Here's the drawing with two shaded views (mm, measured from the low corner). I have some questions. Coordinates: 2 decimals unless noted, no trailing zeros. Order: outer loops, then holes, each group sorted by start corner. A loop starts at its lowest first (then second) coordinate and runs counter-clockwise, first axis right, second up. Notation, with made-up numbers: (77, 88.25) -> (90, 88.25) arc R15 cw to (90, 101.25) -> close; hole circle Ø7 at (80, -4). An arc over 180 degrees is marked (long way). One line per item, written item: value. Start each with the question number.
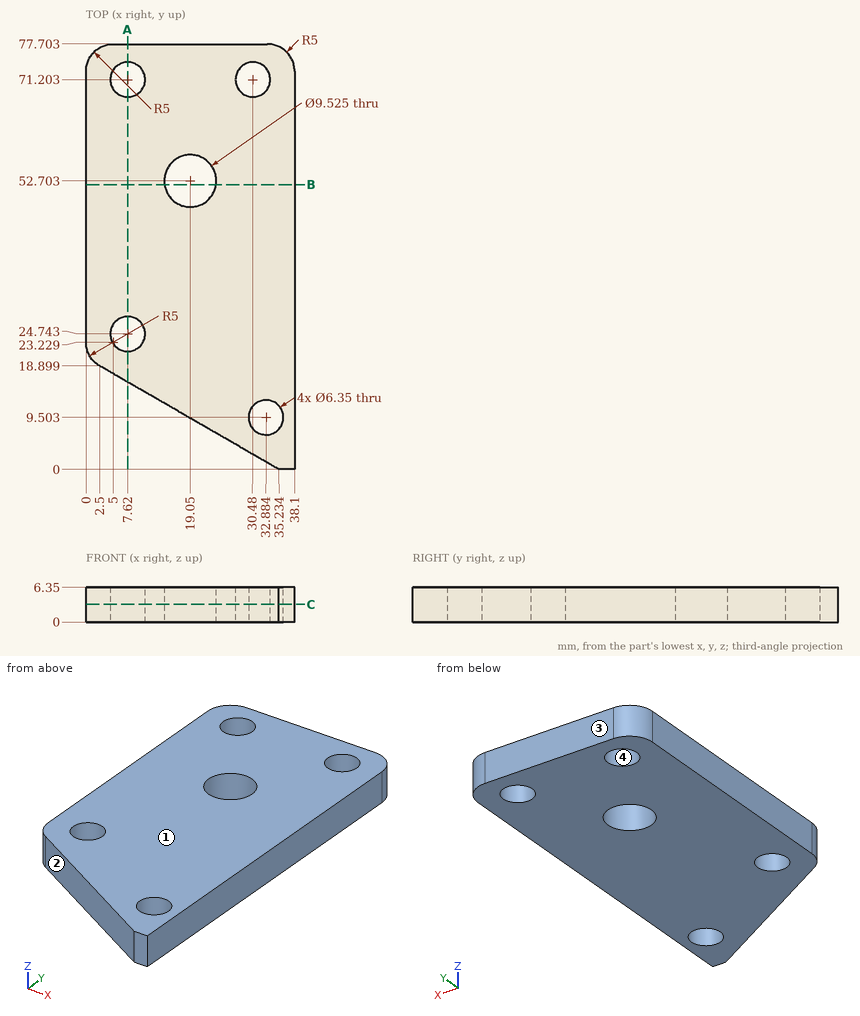
Q1. Imagine slicing it at C-C (z = 3.25). Count the separate pieces of the cut face and the enclosed holes in it, plus the area to 3 significant figures.
Q2. Imagine slicing it at A-A (x = 7.62). Write out the boundary of the cut face in (y, z).
Q3. I need wall thicknesses on line 1 (Y direction, x = 31, z = 1.5) (1 decimal); line 2 (Y direction, x = 7.62, z = 5); line 3 (X direction, y = 26, z = 5.25) (1 decimal). Which ranges of each line are inside material? Lowest first, please.
Q4. If we mould it in two halves opening along Y, with no side actions, what happens to the marked faces 1, 2, 3 and 4? For each: +Y half, -Y half, draft (parallel to the pull), parting line (faces both ways), or undercut.
Q5. Imagine slicing it at B-B (y = 52). Write out the boundary of the cut face in (x, z).
Completed:
1. separate pieces: 1
1. enclosed holes: 5
1. area: 2,390 mm2
2. outline: (15.94, 0) -> (21.57, 0) -> (21.57, 6.35) -> (15.94, 6.35) -> close; (27.92, 0) -> (68.03, 0) -> (68.03, 6.35) -> (27.92, 6.35) -> close; (74.38, 0) -> (77.7, 0) -> (77.7, 6.35) -> (74.38, 6.35) -> close
3. line 1: y = 2.4 to 6.9, 12.1 to 68.1, 74.3 to 77.7
3. line 2: y = 15.94 to 21.57, 27.92 to 68.03, 74.38 to 77.7
3. line 3: x = 0 to 4.7, 10.5 to 38.1
4. face 1: draft
4. face 2: -Y half
4. face 3: +Y half
4. face 4: undercut
5. outline: (0, 0) -> (14.34, 0) -> (14.34, 6.35) -> (0, 6.35) -> close; (23.76, 0) -> (38.1, 0) -> (38.1, 6.35) -> (23.76, 6.35) -> close
